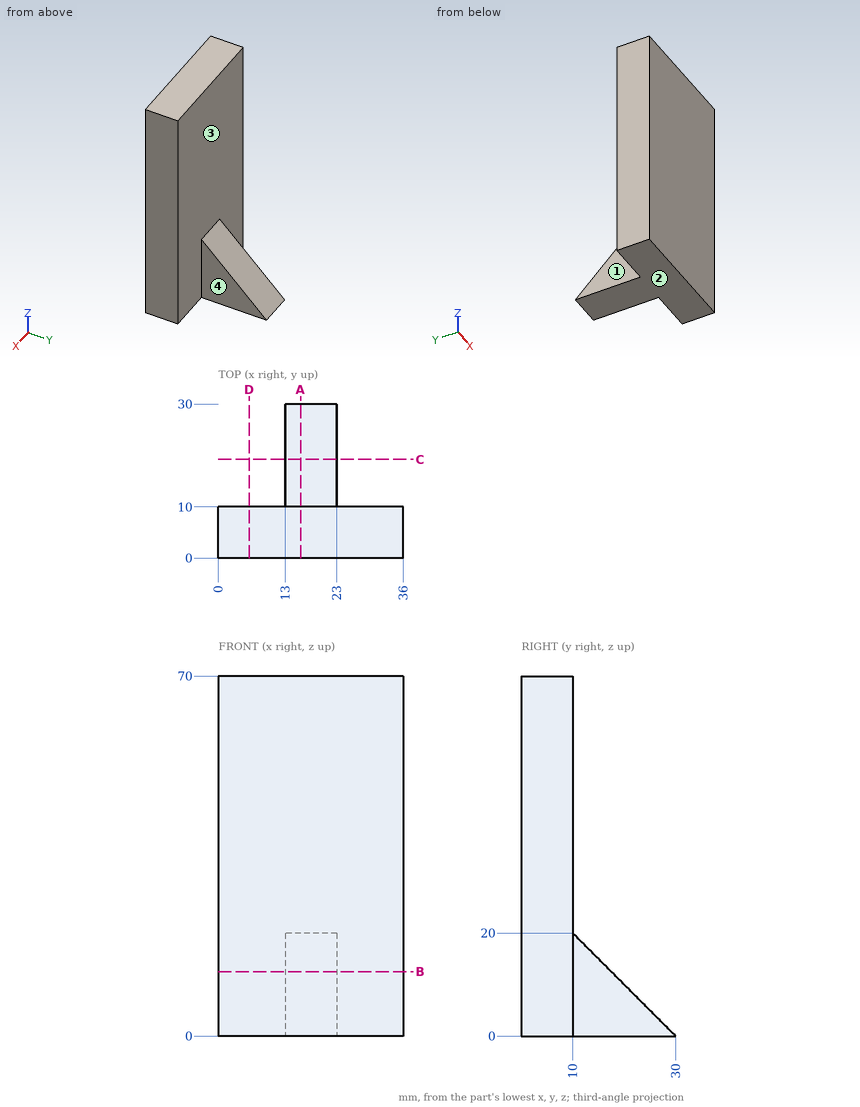
Here's the drawing with two shaded views (mm, measured from the low corner). I have some questions. A direction names the side the tool comes from. Give positions to 0.01 mm unless a question says otherwise; leave off trailing zeros. Loops run counter-clockwise (first coordinate to the right, second up) from the corner with the lowest first, then second, coordinate; pieces in that order, holes last. Notation, with made-up numbers: (40, -36) -> (46, -36) arc R16 ccw to (46, -12) -> close; hole circle Ø3 at (45.25, 30). An arc over 180 degrees is marked (long way). Use one line per item in the form item = value.
1) If we section it at D-D (x = 6): Please give me the cut outline in (y, z), plus the area to 3 significant figures.
Answers:
outline = (0, 0) -> (10, 0) -> (10, 70) -> (0, 70) -> close
area = 700 mm²
2) For the marked faces 1, 2, 3 and 4, which set-ups out of +Z, -Z, +X, -X, +Y, -Y let a thin tool reach every point of the face, with its end or its side?
Answers:
face_1 = +Z, -Z, -X, +Y
face_2 = -Z, +X, -X, +Y, -Y
face_3 = +Z, +Y
face_4 = +Z, -Z, +X, +Y
3) If we section it at A-A (x = 16): Please give me the cut outline in (y, z), plus the area to 3 significant figures.
Answers:
outline = (0, 0) -> (30, 0) -> (10, 20) -> (10, 70) -> (0, 70) -> close
area = 900 mm²
4) If we section it at C-C (y = 19.25): Please give me the cut outline in (x, z), plus the area to 4 significant figures.
Answers:
outline = (13, 0) -> (23, 0) -> (23, 10.75) -> (13, 10.75) -> close
area = 107.5 mm²
5) I need wall thicknesses on line 1 along X through (y, z) = (19.25, 7); line 2 along Y through (x, z) = (7, 48); line 3 along Z through (x, y) = (18.5, 22). Which ranges of each line are inside material? Lowest first, please.
Answers:
line_1 = 13 to 23
line_2 = 0 to 10
line_3 = 0 to 8
6) Will these pins go through, and if not, where does the flat tip stop? pin 1 (16 mm diameter, centred on y = 20.5, z = 15, fed in from +X); pin 2 (10 mm diameter, centred on x = 23, y = 19.5, fed in from +Z); pin 3 (1.5 mm diameter, centred on x = 22, y = 24.5, fed in from +Z); pin 4 (1.5 mm diameter, centred on y = 4.5, z = 54.5, fed in from -X).
Answers:
pin_1 = 23
pin_2 = 15.5
pin_3 = 6.25
pin_4 = 0
7) If we section it at B-B (z = 12.5): Please give me the cut outline in (x, y).
Answers:
outline = (0, 0) -> (36, 0) -> (36, 10) -> (23, 10) -> (23, 17.5) -> (13, 17.5) -> (13, 10) -> (0, 10) -> close
